Job drawing, mm, ordinate dimensions from the low corner. One solid piece. A direction names the side the tool comes from. Give positions to 0.01 mm unless a question says otherwise; leave off trailing zeros. Order: outer loops, then holes, each group sorted by start corner. A loop starts at its lowest first (then second) coordinate and runs counter-clockwise, first axis right, second up.
Item 1: Band-saw the part on A-A on y = 6.35. Count the separate pieces of the cut face and the enclosed holes in it, plus the area to 3 significant figures.
Item 2: Wall check: L1, parallel to X at y = 4.5, z = 18 (1 decimal); L2, parallel to X at y = 9, z = 125.5; L3, parallel to Z at x = 61, y = 1.25. Give the ranges that are in metal, low to high.
Item 3: Flat gauge pins, fed straight in: P1, Ø4, axis at x = 58.5, y = 9, coming from the +Z side; P2, Ø4, axis at x = 116.332, z = 135.128, coming from the +Y side; P3, Ø2, axis at y = 7.5, z = 26.5, coming from the -X side. Where does each tip first touch, or does it go through?
Item 4: Band-saw the part on B-B on x = 90. Give the cut face in (y, z).
Item 5: Which spindle directions (+Z, -Z, +X, -X, +Y, -Y) get a long thin tool onto all of the face, cutting with end or side? Do the marked faces 1 and 2. Say none if no direction does.
Item 6: Band-saw the part on C-C on z = 51. Give the cut face in (x, y).
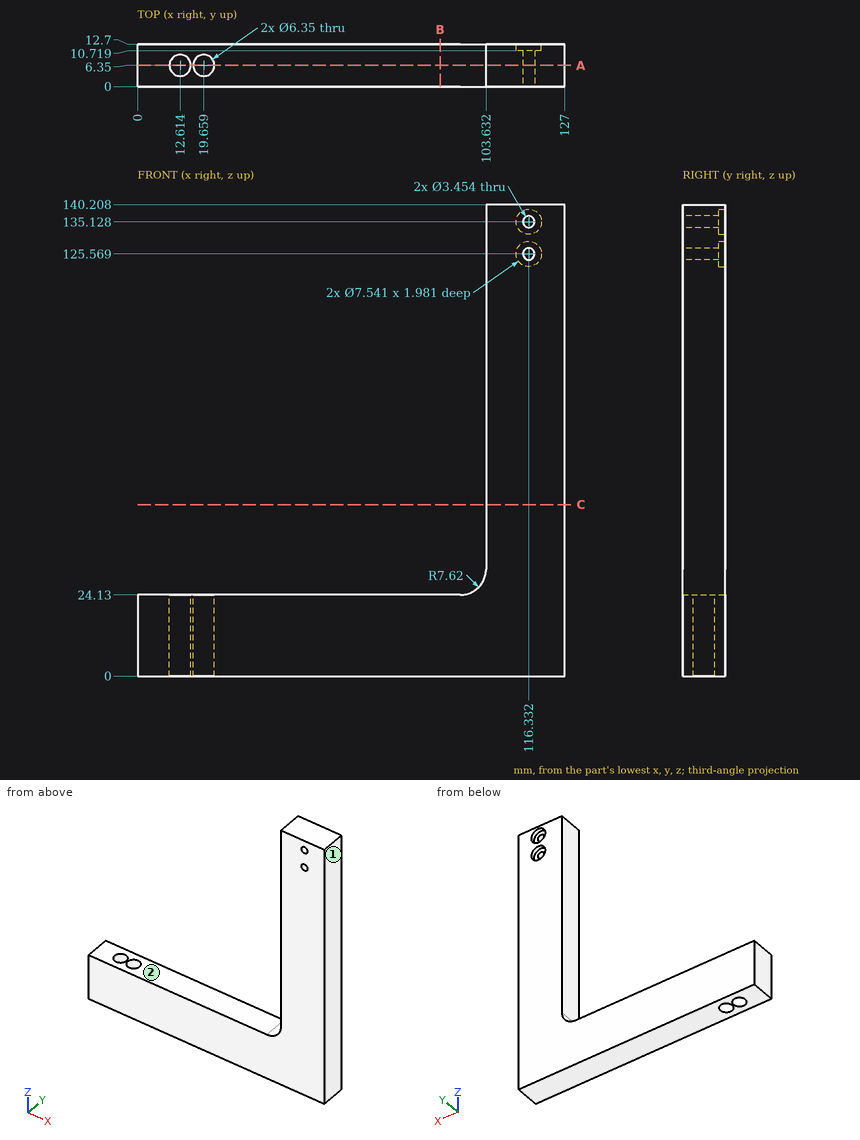
The answers:
1. separate pieces: 3
1. enclosed holes: 2
1. area: 5,460 mm2
2. L1: x = 0 to 10, 15.2 to 17.1, 22.2 to 127
2. L2: x = 103.63 to 114.61, 118.06 to 127
2. L3: z = 0 to 24.13
3. P1: stops at z = 24.13
3. P2: stops at y = 10.72
3. P3: stops at x = 100.37
4. outline: (0, 0) - (12.7, 0) - (12.7, 24.13) - (0, 24.13) - close
5. face 1: +Z, -Z, +X, +Y, -Y
5. face 2: +Z, -X, +Y, -Y
6. outline: (103.63, 0) - (127, 0) - (127, 12.7) - (103.63, 12.7) - close
